Here's the drawing with two shaded views (mm, measured from the low corner). I have some questions. A direction names the side the tool comes from. Give positions to 0.01 mm unless a question says otherwise; leave off trailing zeros. Write each loop counter-clockwise with the first axis right and the second up, starting at its lowest first coordinate (ties: lowest second). Pieces come first, ordered by that corner, then holes.
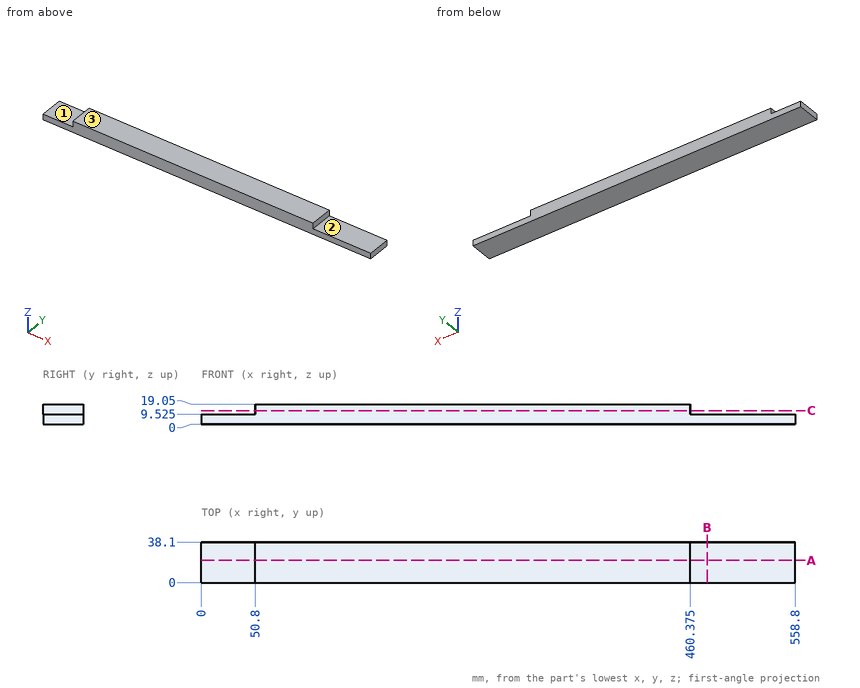
(1) Imagine slicing it at B-B, the plane x = 476. Write out the boundary of the cut face in (y, z) (3 decimals).
Returned:
outline: (0, 0) - (38.1, 0) - (38.1, 9.525) - (0, 9.525) - close
(2) If I drill on L1, parallel to X at y = 23, z = 13 (3 decimals); L2, parallel to Z at x = 532.5, y = 21.5 (3 decimals), over which ranges is the centre line in solid material (lowest first)?
Returned:
L1: x = 50.8 to 460.375
L2: z = 0 to 9.525
(3) Imagine slicing it at C-C, the plane z = 12.75. Write out the boundary of the cut face in (x, y) (3 decimals).
Returned:
outline: (50.8, 0) - (460.375, 0) - (460.375, 38.1) - (50.8, 38.1) - close
(4) For the marked faces 1, 2 and 3, which set-ups out of +Z, -Z, +X, -X, +Y, -Y let a thin tool reach every point of the face, with its end or its side?
Returned:
face 1: +Z, -X, +Y, -Y
face 2: +Z, +X, +Y, -Y
face 3: +Z, +X, -X, +Y, -Y
(5) Imagine slicing it at A-A, the plane y = 21. Write out the boundary of the cut face in (x, z) (3 decimals), plus the area to 3 significant figures.
Returned:
outline: (0, 0) - (558.8, 0) - (558.8, 9.525) - (460.375, 9.525) - (460.375, 19.05) - (50.8, 19.05) - (50.8, 9.525) - (0, 9.525) - close
area: 9,220 mm2
(6) Will these pins go through, and if not, where does the flat tip stop? P1, Ø3, axis at y = 5, z = 13, coming from the -X side; P2, Ø11.5, axis at x = 30.5, y = 22, coming from the +Z side (3 decimals); P3, Ø5, axis at y = 19, z = 16.5, coming from the +X side (3 decimals).
Returned:
P1: stops at x = 50.8
P2: stops at z = 9.525
P3: stops at x = 460.375
